Geometry: final body of the model. Coordinates: model frame, mm. Face numbers are marked on the shaded views. A direction names the side the tool comes from. Give positions to 0.01 mm unless a question says otherwise; leave off trailing zeros. Write each loop counter-clockwise with the first axis right and the second up, starting at its lowest first coordinate (ties: lowest second). Pieces come first, ordered by that corner, then holes.
Q1. Pin query (flat end, axial travel): pin 1 Ø2 at (x, y) = (2.5, -3) entering from -Z; pin 2 Ø2 at (x, z) = (-14, -4) entering from -Y; pin 3 Ø1.5 at (x, z) = (13.5, 2.5) entering from +Y. Return the tip coordinate at first contact, or that it passes through.
Q2. Section A-A (z = 0). Return the cut outline in (x, y), plus the area to 3 significant figures.
Q3. Line query: line 1 (X direction, y = 5.5, z = 3.5); line 2 (Z direction, x = -4, y = -0.25); line 3 (X direction, y = -2.25, z = -1.25). Output: solid intervals per line, ascending.
Q4. Section C-C (x = 21.5). Return the cut outline in (y, z), plus the area to 3 significant figures.
Q5. Reachability of the marked faces 1, 2 and 3 from +Z, -Z, +X, -X, +Y, -Y: full face, straight path, thin tool, end or side. Return the list, or none.
Q6. Section D-D (x = -24). Return the cut outline in (y, z).
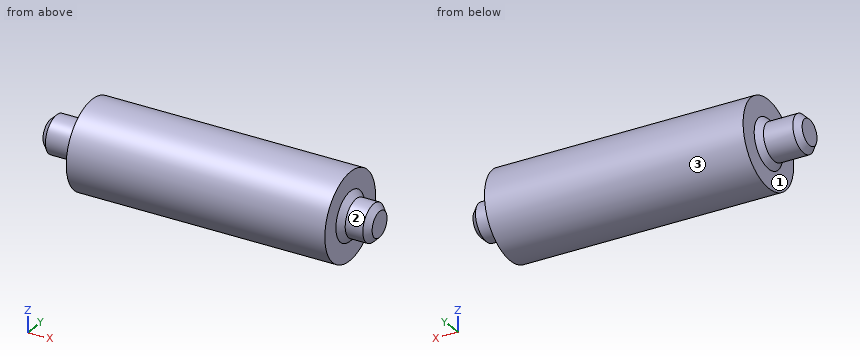
from build123d import *

# Parameters (mm, degrees)
CHAMFER1_SIZE = 1
CHAMFER2_SIZE = 1


with BuildPart() as part:
    # Sketch1 → Revolve1 (revolve)
    with BuildSketch(Plane.XY):
        Polygon((-28.142857143, 0), (-28.142857143, 3.18), (-21.142857143, 3.18), (-21.142857143, 7.43), (22.857142857, 7.43), (22.857142857, 3.18), (27.857142857, 3.18), (27.857142857, 0), align=None)
    revolve(axis=Axis((-28.142857143, 0, 0), (1, 0, 0)))

    # Chamfer1
    chamfer1_edges = [part.edges().sort_by_distance(p)[0] for p in [
        (27.857142857, -3.18, 0),
        (-28.142857143, -3.18, 0),
    ]]
    chamfer(chamfer1_edges, length=CHAMFER1_SIZE)

    # Chamfer2
    chamfer2_edges = [part.edges().sort_by_distance(p)[0] for p in [
        (22.857142857, -3.18, 0),
        (-21.142857143, -3.18, 0),
    ]]
    chamfer(chamfer2_edges, length=CHAMFER2_SIZE)


solid = part.part
Computed:
1. pin 1: stops at z = -7.16
1. pin 2: stops at y = -6.8
1. pin 3: stops at y = 7.22
2. outline: (-28.14, -2.18) - (-27.14, -3.18) - (-22.14, -3.18) - (-21.14, -4.18) - (-21.14, -7.43) - (22.86, -7.43) - (22.86, -4.18) - (23.86, -3.18) - (26.86, -3.18) - (27.86, -2.18) - (27.86, 2.18) - (26.86, 3.18) - (23.86, 3.18) - (22.86, 4.18) - (22.86, 7.43) - (-21.14, 7.43) - (-21.14, 4.18) - (-22.14, 3.18) - (-27.14, 3.18) - (-28.14, 2.18) - close
2. area: 730 mm2
3. line 1: x = -21.14 to 22.86
3. line 2: z = -7.43 to 7.43
3. line 3: x = -27.75 to 27.46
4. outline: circle Ø14.86 at (0, 0)
4. area: 173 mm2
5. face 1: -X
5. face 2: +X
5. face 3: +X, -X
6. outline: circle Ø6.36 at (0, 0)
